Source: three-view drawing plus pictorial views. Frame: mm from the lowest corner of the part. A direction names the side the tool comes from. Give positions to 0.01 mm unless a question says otherwise; leave off trailing zeros. Loops run counter-clockwise (first coordinate to the right, second up) from the corner with the lowest first, then second, coordinate; pieces in that order, holes last. Notation, with made-up numbers: M 65.25,38 L 98.25,38 A18 cw 98.25,49 Z; hole C 15.25,85 d2. An arc over 180 degrees is marked long. Answer as a JSON object with one key per item and string values. Group by question number.
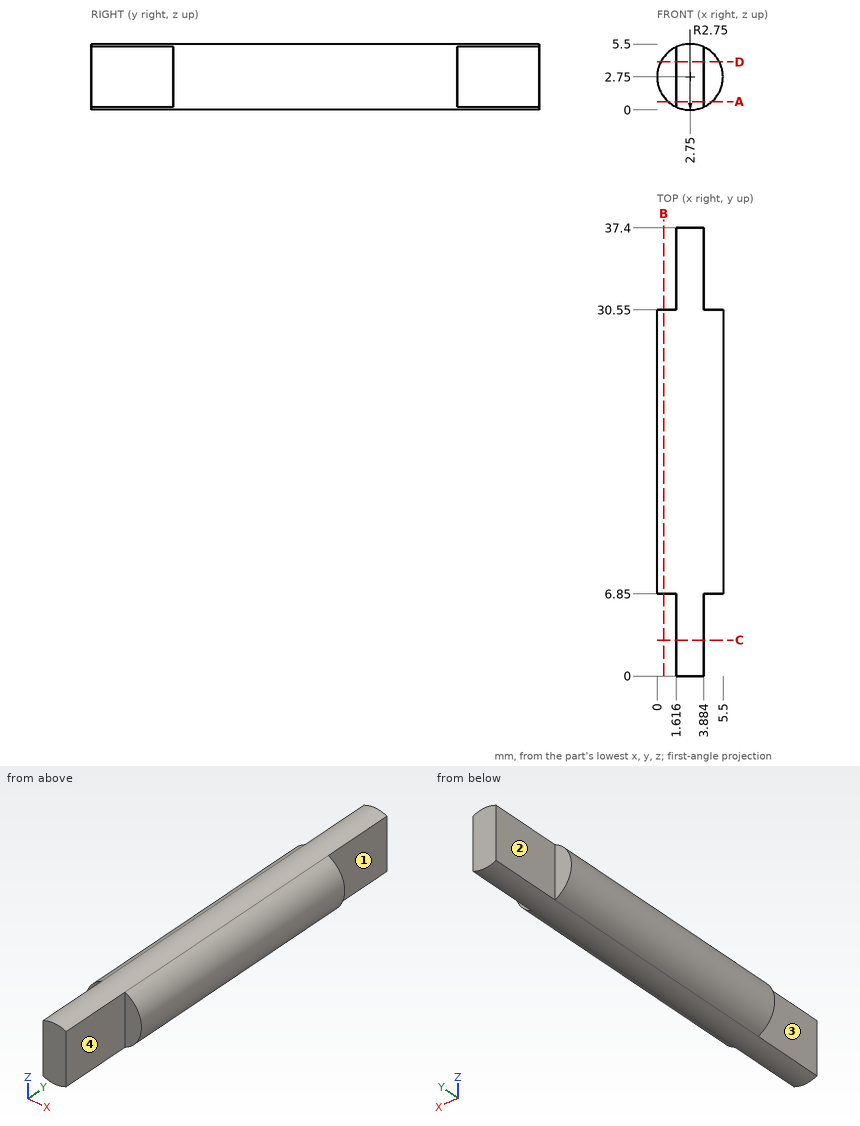
1. Section D-D (z = 4). Output: boundary loops of the cut face in (x, y).
2. Reachability of the marked faces 1, 2, 3 and 4 from +Z, -Z, +X, -X, +Y, -Y: full face, straight path, thin tool, end or side. Return the list, or none.
3. Material intervals for L1, parallel to Y at x = 0.2, z = 2.8; L2, parallel to Z at x = 2.9, y = 35; L3, parallel to X at y = 35.5, z = 3.2, sorted ascending.
4. First-contact query: P1, Ø0.8, axis at x = 1, z = 2.5, coming from the +Y side; P2, Ø2, axis at x = 1.5, y = 28.5, coming from the -Z side; P3, Ø1.5, axis at y = 32.5, z = 4, coming from the +X side. Flat tips, straight axial feed; report the tip coordinate or a pass-through.
5. Section C-C (y = 3). Output: boundary loops of the cut face in (x, z).
6. Section B-B (x = 0.55). Output: boundary loops of the cut face in (y, z), then the cut area to 3 significant figures.
7. Section A-A (z = 0.7). Output: boundary loops of the cut face in (x, y).
Geometry results:
{
 "1": {"outline": "M 0.3,6.85 L 1.62,6.85 L 1.62,0 L 3.88,0 L 3.88,6.85 L 5.2,6.85 L 5.2,30.55 L 3.88,30.55 L 3.88,37.4 L 1.62,37.4 L 1.62,30.55 L 0.3,30.55 Z"},
 "2": {"face 1": "+Z, -Z, +X, +Y", "face 2": "+Z, -Z, -X, +Y", "face 3": "+Z, -Z, -X, -Y", "face 4": "+Z, -Z, +X, -Y"},
 "3": {"L1": "6.85 to 30.55", "L2": "0 to 5.5", "L3": "1.62 to 3.88"},
 "4": {"P1": "y = 30.55", "P2": "z = 0.01", "P3": "x = 3.88"},
 "5": {"outline": "M 1.62,0.24 A2.75 ccw 3.88,0.24 L 3.88,5.26 A2.75 ccw 1.62,5.26 Z"},
 "6": {"outline": "M 6.85,1.1 L 30.55,1.1 L 30.55,4.4 L 6.85,4.4 Z", "area": "78.2 mm2"},
 "7": {"outline": "M 0.92,6.85 L 1.62,6.85 L 1.62,0 L 3.88,0 L 3.88,6.85 L 4.58,6.85 L 4.58,30.55 L 3.88,30.55 L 3.88,37.4 L 1.62,37.4 L 1.62,30.55 L 0.92,30.55 Z"}
}
